Could you check a few things on this drawing? It's one solid part, dimensions in mm from its lowest x, y, z. A direction names the side the tool comes from. Give positions to 0.01 mm unless a question says otherwise; leave off trailing zeros. Loops run counter-clockwise (first coordinate to the right, second up) from the corner with the lowest first, then second, coordinate; pieces in that order, holes last.
1. Imagine slicing it at B-B (x = 20). List the corners of the cut face in (y, z) for me, plus the area to 3 significant figures.
2. Imagine slicing it at C-C (y = 6.5). List the corners of the cut face in (x, z) for me, plus the area to 3 significant figures.
3. Thinking about a two-plate mould opening in X: for the marked faces 6, 7 and 8, which applies, +X half, -X half, draft (parallel to the pull), parting line (faces both ways), or undercut?
4. For the marked faces 1, 2, 3, 4 and 5, which set-ups out of +Z, -Z, +X, -X, +Y, -Y let a thin tool reach every point of the face, with its end or its side?
5. I need wall thicknesses on line 1 along X through (y, z) = (8, 8.25); line 2 along Y through (x, z) = (20, 6.5); line 3 along X through (y, z) = (35.5, 0.75). Which ranges of each line are inside material? Lowest first, please.
6. Imagine slicing it at D-D (z = 2.25). List the corners of the cut face in (x, y) for me (3 decimals).
7. For P1, Ø2, axis at x = 31, z = 1.5, coming from the -Y side; P2, Ø1, axis at x = 2.5, z = 3.5, coming from the +Y side; P3, Ø5, axis at y = 29.5, z = 7.5, coming from the +X side; P4, Ø5, axis at y = 30, z = 3, coming from the -X side, each with a flat end and sliding along its axis, tell me the tip position at first contact or that it passes through.
8. Imagine slicing it at A-A (z = 8.5). List the corners of the cut face in (x, y) for me.
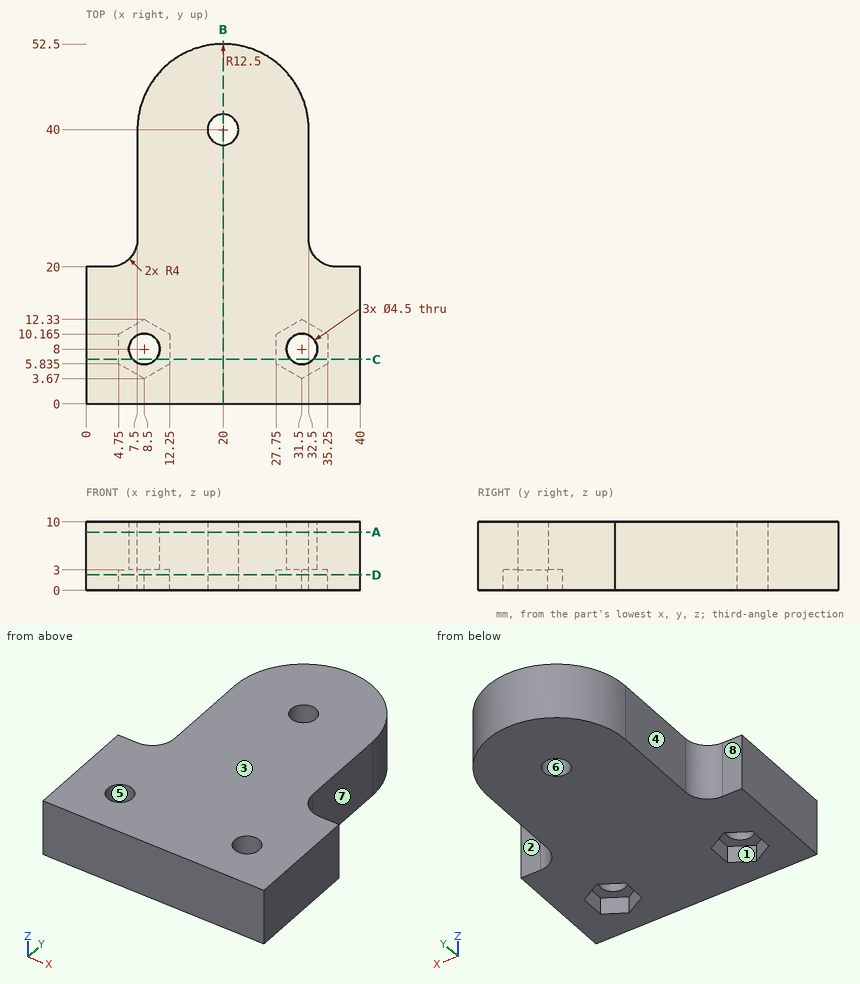
Derived:
1. outline: (0, 0) - (37.75, 0) - (37.75, 10) - (0, 10) - close; (42.25, 0) - (52.5, 0) - (52.5, 10) - (42.25, 10) - close
1. area: 480 mm2
2. outline: (0, 0) - (4.75, 0) - (4.75, 3) - (6.82, 3) - (6.82, 10) - (0, 10) - close; (10.18, 3) - (12.25, 3) - (12.25, 0) - (27.75, 0) - (27.75, 3) - (29.82, 3) - (29.82, 10) - (10.18, 10) - close; (33.18, 3) - (35.25, 3) - (35.25, 0) - (40, 0) - (40, 10) - (33.18, 10) - close
2. area: 308 mm2
3. face 6: undercut
3. face 7: +X half
3. face 8: draft
4. face 1: -Z
4. face 2: +Z, -Z, +X, +Y
4. face 3: +Z, +X, -X, +Y, -Y
4. face 4: +Z, -Z, -X, +Y
4. face 5: +Z, -Z
5. line 1: x = 0 to 6.25, 10.75 to 29.25, 33.75 to 40
5. line 2: y = 0 to 37.75, 42.25 to 52.5
5. line 3: x = 7.5 to 32.5
6. outline: (0, 0) - (40, 0) - (40, 20) - (36.5, 20) arc R4 cw to (32.5, 24) - (32.5, 40) arc R12.5 ccw to (7.5, 40) - (7.5, 24) arc R4 cw to (3.5, 20) - (0, 20) - close; hole (4.75, 5.835) - (8.5, 3.67) - (12.25, 5.835) - (12.25, 10.165) - (8.5, 12.33) - (4.75, 10.165) - close; hole circle Ø4.5 at (20, 40); hole (27.75, 5.835) - (31.5, 3.67) - (35.25, 5.835) - (35.25, 10.165) - (31.5, 12.33) - (27.75, 10.165) - close
7. P1: stops at y = 0
7. P2: stops at y = 20
7. P3: stops at x = 32.5
7. P4: stops at x = 7.5
8. outline: (0, 0) - (40, 0) - (40, 20) - (36.5, 20) arc R4 cw to (32.5, 24) - (32.5, 40) arc R12.5 ccw to (7.5, 40) - (7.5, 24) arc R4 cw to (3.5, 20) - (0, 20) - close; hole circle Ø4.5 at (8.5, 8); hole circle Ø4.5 at (20, 40); hole circle Ø4.5 at (31.5, 8)
